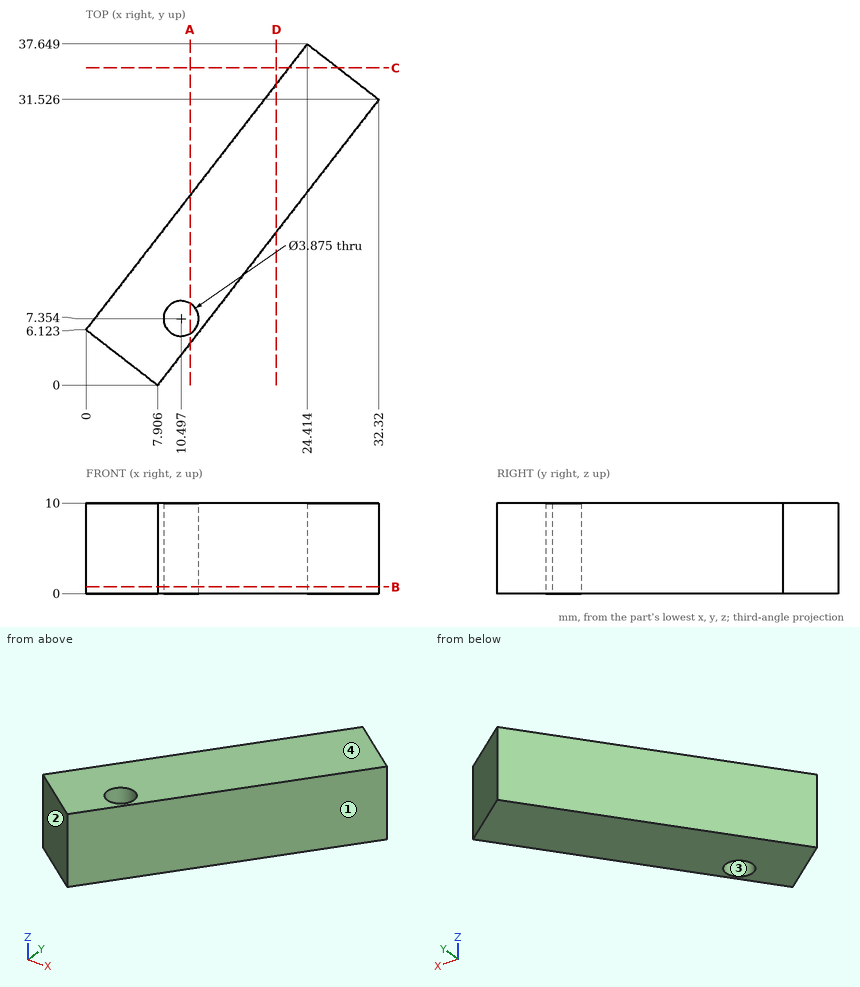
Design review of the part shown in the three views and the two pictorial views. Dimensions are in mm from the part's minimum x, y and z. Give positions to 0.01 mm unless a question says otherwise; leave off trailing zeros. Loops run counter-clockwise (first coordinate to the right, second up) from the corner with the lowest first, then second, coordinate; pieces in that order, holes last. Notation, with made-up numbers: (-40, 11.25) - (14, 11.25) arc R28 ccw to (14, 31.25) - close; hole circle Ø9 at (66, 83.5). An arc over 180 degrees is marked (long way). Write item = value, one per line.
1) Clearance check with flat-ended pins moving along their axes: pin 1 Ø5 at (x, z) = (16, 5) entering from -Y (1 decimal); pin 2 Ø1.5 at (x, z) = (5.5, 3.5) entering from +Y (1 decimal); pin 3 Ø3 at (x, z) = (21.5, 4.5) entering from +Y (1 decimal); pin 4 Ø1.5 at (y, z) = (6, 4.5) entering from -X. State where each tip first meets the part, or that it passes through.
Result sheet:
pin_1 = 7.2
pin_2 = 14.2
pin_3 = 35.8
pin_4 = 0
2) Take a section at A-A on x = 11.5. State the section outline as (y, z) points, and give its area (3 significant figures).
Result sheet:
outline = (4.64, 0) - (5.7, 0) - (5.7, 10) - (4.64, 10) - close; (9.01, 0) - (20.97, 0) - (20.97, 10) - (9.01, 10) - close
area = 130 mm2
3) Take a section at D-D on x = 21. State the section outline as (y, z) points, and give its area (3 significant figures).
Result sheet:
outline = (16.91, 0) - (33.24, 0) - (33.24, 10) - (16.91, 10) - close
area = 163 mm2
4) To check wall thickness, follow line 1 (X direction, y = 8.5, z = 3) (1 decimal); line 2 (X direction, y = 6.5, z = 9.25) (1 decimal); line 3 (Y direction, x = 7, z = 4.75) (1 decimal). State the ranges of each line that lie inside material, in increasing order.
Result sheet:
line_1 = 1.8 to 8.9, 12.1 to 14.5
line_2 = 0.3 to 8.8, 12.2 to 12.9
line_3 = 0.7 to 15.2
5) Take a section at B-B on z = 0.75. State the section outline as (x, y) points (1 decimal).
Result sheet:
outline = (0, 6.1) - (7.9, 0) - (32.3, 31.5) - (24.4, 37.6) - close; hole circle Ø3.9 at (10.5, 7.4)
6) Draft analysis for pull direction X (two halves, no side actions). For the marked faces 1, 2, 3 and 4, state which applies: +X half, -X half, draft (parallel to the pull), parting line (faces both ways), or undercut.
Result sheet:
face_1 = +X half
face_2 = -X half
face_3 = undercut
face_4 = draft
7) Take a section at C-C on y = 35. State the section outline as (x, z) points, and give its area (3 significant figures).
Result sheet:
outline = (22.36, 0) - (27.83, 0) - (27.83, 10) - (22.36, 10) - close
area = 54.7 mm2
